Read the model definition and answer for the solid it produces. Units are mm, in the model's axes. A direction names the side the tool comes from. Coordinates: 2 decimals unless noted, no trailing zeros. Write each loop counter-clockwise with the first axis right and the second up, starting at its lowest first coordinate (ties: lowest second). Pieces come first, ordered by that corner, then holes.
Autodesk Inventor part; units mm, degrees
ref_plane "YZ Plane" through (0, 0, 0) normal (1, 0, 0) x (0, 1, 0)
ref_plane "XZ Plane" through (0, 0, 0) normal (0, 1, 0) x (-1, 0, 0)
ref_plane "XY Plane" through (0, 0, 0) normal (0, 0, 1) x (1, 0, 0)
sketch "Эскиз1" plane through (0, 0, 0) normal (0, 1, 0) x (-1, 0, 0)
  circle A0 centre (0, 0) radius 30
  dimension "d0" = 60
extrude "Выдавливание1" add sketch "Эскиз1" along normal blind 15
sketch "Эскиз3" plane through (0, 0, 0) normal (0, -1, 0) x (1, 0, 0)
  circle A0 centre (0, 0) radius 20
  line L0 (0, 0) -> (30, 0) construction
  line L1 (0, 0) -> (30, 0) construction
  line L2 (0, 0) -> (30, 0) construction
  line L3 (0, 0) -> (30, 0) construction
  line L4 (0, 0) -> (14.1421, 14.1421)
  line L5 (0, 0) -> (20, 0) construction
  line L6 (0, 0) -> (14.1421, -14.1421)
  line L7 (0, 0) -> (-14.1421, 14.1421)
  line L8 (0, 0) -> (20, 0) construction
  line L9 (0, 0) -> (-14.1421, -14.1421)
  line L10 (0, 0) -> (20, 0) construction
  circle A1 centre (14.1421, 14.1421) radius 7.5
  circle A2 centre (14.1421, -14.1421) radius 7.5
  circle A3 centre (-14.1421, -14.1421) radius 7.5
  circle A4 centre (-14.1421, 14.1421) radius 7.5
  point P0 (-8.7707, -17.9743)
  point P1 (-16.2945, -11.5969)
  point P2 (-8.7707, 17.9743)
  point P3 (-16.2945, 11.5969)
  point P4 (11.5969, -16.2945)
  point P5 (17.9743, -8.7707)
  point P6 (17.995, 8.7282)
  point P7 (11.5862, 16.3021)
  point P8 (18.357, 7.9385)
  point P9 (7.9385, 18.357)
  point P10 (-7.9385, 18.357)
  point P11 (-18.357, 7.9385)
  point P12 (-18.357, -7.9385)
  point P13 (-7.9385, -18.357)
  point P14 (7.9385, -18.357)
  point P15 (18.357, -7.9385)
  dimension "d26" = 40
  dimension "d62" = 20
  dimension "d63" = 45
  dimension "d64" = 20
  dimension "d65" = 20
  dimension "d66" = 135
  dimension "d67" = 20
  dimension "d68" = 135
  dimension "d69" = 15
  dimension "d70" = 15
  dimension "d71" = 15
  dimension "d72" = 15
sketch "Эскиз4" plane through (0, 15, 0) normal (0, 1, 0) x (1, 0, 0)
  circle A0 centre (0, 0) radius 15
  dimension "d41" = 30
extrude "Выдавливание3" add sketch "Эскиз4" along normal blind 35
sketch "Эскиз5" plane through (0, 15, 0) normal (0, 1, 0) x (1, 0, 0)
  line L0 (0, 0) -> (0, -25)
  arc A0 (20, 0) -> (20, 0) centre (0, 0) ccw
  line L1 (0, 0) -> (25, 0)
  line L2 (0, 0) -> (0, 25)
  line L3 (0, 0) -> (-25, 0)
  dimension "d44" = 25
  dimension "d45" = 25
  dimension "d46" = 25
  dimension "d47" = 25
hole "Отверстие3" at (0, 15, 25) at (-25, 15, 0) at (0, 15, -25) at (25, 15, 0) direction (0, -1, 0) diameter 6 end through all
extrude "Выдавливание4" add sketch "Эскиз3" along normal blind 30
properties part number "Крепление Барабана2" material "Сталь, литейная"
Item 1: The part is cut by section B-B (y = 8.5). Give the vertices of the cut face in (x, z).
Item 2: The part is cut by section C-C (y = -16). Give the vertices of the cut face in (x, z), and give its area (3 significant figures).
Item 3: Determine the mould class of faces 1 (the cylindrical face through (0, 7, -28)), 2 (the cylindrical face through (0, -15, -20)), 3 (the cylindrical face through (-14.985, 32.255, 0.66)), 4 (the flat face through (0, -30, 0)) for opening direction Z: +Z half, -Z half, draft (parallel to the pull), parting line (faces both ways), or undercut.
Item 4: For faces 5 (the flat face through (2.4, 0, 20.1)), 6 (the cylindrical face through (0, -15, 20)), 7 (the flat face through (-6, 15, 14)), determine the directions among +Z, -Z, +X, -X, +Y, -Y from which every point of the face is accessible in a straight line to the end or side of a thin tool.
Item 5: Find the intervals of material crossed by probe 1 along Z at (x, y) = (0, 12); probe 2 along Y at (x, z) = (15.5, -6.5); probe 3 along Y at (x, z) = (-26.5, -6), in increasing order.
Item 6: The part is cut by section A-A (z = 0). Give the vertices of the cut face in (x, y), and give its area (3 significant figures).
Item 7: The part is cut by section D-D (x = 25). Give the vertices of the cut face in (y, z), and give its area (3 significant figures).
Item 8: Given pin 1 (5 mm diameter, centred on x = 8, y = 29.5, fed in from -Z); pin 2 (5.5 mm diameter, centred on x = 0, z = 25, fed in from -Y); pin 3 (10 mm diameter, centred on y = -20.5, z = 2, fed in from +X); pin 4 (12 mm diameter, centred on x = 7.5, y = -8.5, fed in from -Z), each flat-ended and moving along its own axis, determine where each tip first touches the part or whether it passes through.
Answer:
1. outline: circle Ø60 at (0, 0); hole circle Ø6 at (-25, 0); hole circle Ø6 at (0, -25); hole circle Ø6 at (0, 25); hole circle Ø6 at (25, 0)
2. outline: (-18.36, -7.94) arc R7.5 ccw (long way) to (-7.94, -18.36) arc R20 ccw to (7.94, -18.36) arc R7.5 ccw (long way) to (18.36, -7.94) arc R20 ccw to (18.36, 7.94) arc R7.5 ccw (long way) to (7.94, 18.36) arc R20 ccw to (-7.94, 18.36) arc R7.5 ccw (long way) to (-18.36, 7.94) arc R20 ccw to start
2. area: 1,640 mm2
3. face 1: undercut
3. face 2: -Z half
3. face 3: parting line
3. face 4: draft
4. face 5: -Y
4. face 6: +Z, -Y
4. face 7: +Y
5. probe 1: z = -30 to -28, -22 to 22, 28 to 30
5. probe 2: y = -30 to 15
5. probe 3: y = 0 to 15
6. outline: (-30, 0) - (-28, 0) - (-28, 15) - (-30, 15) - close; (-22, 0) - (-20, 0) - (-20, -30) - (20, -30) - (20, 0) - (22, 0) - (22, 15) - (15, 15) - (15, 50) - (-15, 50) - (-15, 15) - (-22, 15) - close; (28, 0) - (30, 0) - (30, 15) - (28, 15) - close
6. area: 2,970 mm2
7. outline: (0, -16.58) - (15, -16.58) - (15, -3) - (0, -3) - close; (0, 3) - (15, 3) - (15, 16.58) - (0, 16.58) - close
7. area: 407 mm2
8. pin 1: stops at z = -13.96
8. pin 2: passes through
8. pin 3: stops at x = 20
8. pin 4: stops at z = -21.61
